Autodesk Inventor part; units mm, degrees
ref_plane "YZ Plane" through (0, 0, 0) normal (1, 0, 0) x (0, 1, 0)
ref_plane "XZ Plane" through (0, 0, 0) normal (0, 1, 0) x (-1, 0, 0)
ref_plane "XY Plane" through (0, 0, 0) normal (0, 0, 1) x (1, 0, 0)
sketch "Sketch1" plane through (0, 0, 0) normal (1, 0, 0) x (0, 1, 0)
  line L0 (0.68, 4.039) -> (1, 3.883)
  line L1 (1, 3.883) -> (1, -2.361)
  line L2 (1.16, -3.161) -> (1.41, -3.161)
  line L3 (1.51, -3.261) -> (1.51, -3.861)
  line L4 (1.41, -3.961) -> (0, -3.961)
  line L5 (0, -3.961) -> (0, 3.961)
  arc A0 (1.51, -3.261) -> (1.41, -3.161) centre (1.41, -3.261) ccw
  arc A1 (1.41, -3.961) -> (1.51, -3.861) centre (1.41, -3.861) ccw
  line L6 (0.68, 4.039) -> (0.476, 4.039)
  line L7 (0.476, 4.039) -> (0, 3.961)
  line L8 (1.16, -3.161) -> (1, -3.001)
  arc A2 (1, -2.361) -> (0.85, -2.511) centre (1, -2.511) ccw
  line L9 (0.85, -2.511) -> (0.85, -2.851)
  arc A3 (0.85, -2.851) -> (1, -3.001) centre (1, -2.851) ccw
  point P0 (0, 0)
  point P1 (1.51, -3.161)
  point P2 (1.51, -3.961)
  point P3 (0, 0)
  dimension "d0" = 2
  dimension "d2" = 3.02
  dimension "d4" = 1.36
  dimension "d6" = 0.8
  dimension "d8" = 0.1
  dimension "d9" = 0.156
  dimension "d11" = 8
  dimension "d12" = 0.952
  dimension "d13" = 0.078
  dimension "d14" = 2.32
  dimension "d15" = 135
  dimension "d16" = 0.8
  dimension "d17" = 1.7
revolve "Revolution1" add sketch "Sketch1" angle 360 about axis through (0, 0, -3.961) along (0, 0, 1)
properties part number "Pin_Headed-2x8mm" material "Stainless Steel"
Read the model definition and answer for the solid it produces. Units are mm, in the model's axes. A direction names the side the tool comes from. Round coordinates to 2 decimals unless told otherwise and drop trailing zeros. Order: outer loops, then holes, each group sorted by start corner. A loop starts at its lowest first (then second) coordinate and runs counter-clockwise, first axis right, second up.
1) The mould has two halves that part along Y. Classify faces 1 (the face through (0, 0, -3.961)), 2 (the face through (-0.83, -0.18, -2.68)), 3 (the face through (0.029, -0.006, 3.966)): released by +Y, released by -Y, zero draft, split by the parting line, or undercut.
2) A flat-ended cylindrical pin translates along its axis: pin 1 (1 mm diameter, centred on x = -1, z = 1, fed in from -Y). Find the tip coordinate at first contact, or state that the pin passes through.
3) The part is cut by section A-A on z = 1. Write down the section's boundary in (x, y), plus the area to 3 significant figures.
4) Straight lines are drawn through the part: L1, parallel to Y at x = 0.05, z = -2.5; L2, parallel to Z at x = -0.6, y = -0.75; L3, parallel to X at y = -0.05, z = 0. For each, find the intervals that lie inside material, in ascending order.
5) For faces 4 (the face through (-1, 0, 1)), 5 (the face through (1.497, -0.197, -3.565)), determine the directions among +Z, -Z, +X, -X, +Y, -Y from which every point of the face is accessible in a straight line to the end or side of a thin tool.
Resolved:
1. face 1: zero draft
1. face 2: split by the parting line
1. face 3: undercut
2. pin 1: stops at y = -0.87
3. outline: circle Ø2 at (0, 0)
3. area: 3.14 mm2
4. L1: y = -0.85 to 0.85
4. L2: z = -3.96 to -3, -2.37 to 3.9
4. L3: x = -1 to 1
5. face 4: +Z
5. face 5: +Z, -Z
